Build history of the part. All positions in model axes, mm. Coordinates: 2 decimals unless noted, no trailing zeros. Write each loop counter-clockwise with the first axis right and the second up, starting at its lowest first coordinate (ties: lowest second). Pieces come first, ordered by that corner, then holes.
```python
from build123d import *

# Parameters (mm, degrees)
SKETCH1_W           = 288
SKETCH1_H           = 348
BOSS_EXTRUDE1_DEPTH = 25
SKETCH2_W           = 220
SKETCH2_H           = 25
SKETCH2_W_2         = 25
SKETCH2_H_2         = 280
CUT_EXTRUDE5_DEPTH  = 25


with BuildPart() as part:
    # Sketch1 → Boss-Extrude1 (new body)
    with BuildSketch(Plane(origin=(0, 0, 0), x_dir=(1, 0, 0), z_dir=(0, 1, 0))):
        with Locations((111.777306141, 159.011164947)):
            Rectangle(SKETCH1_W, SKETCH1_H)
    extrude(amount=BOSS_EXTRUDE1_DEPTH)

    # Sketch2 → Cut-Extrude5 (cut)
    with BuildSketch(Plane(origin=(0, 0, 0), x_dir=(1, 0, 0), z_dir=(0, 1, 0))):
        with Locations((111.777306141, 314.511164947)):
            Rectangle(SKETCH2_W, SKETCH2_H)
        with Locations((111.777306141, 3.511164947)):
            Rectangle(SKETCH2_W, SKETCH2_H)
        with Locations((237.277306141, 159.011164947)):
            Rectangle(SKETCH2_W_2, SKETCH2_H_2)
    extrude(amount=CUT_EXTRUDE5_DEPTH, mode=Mode.SUBTRACT)


solid = part.part
```
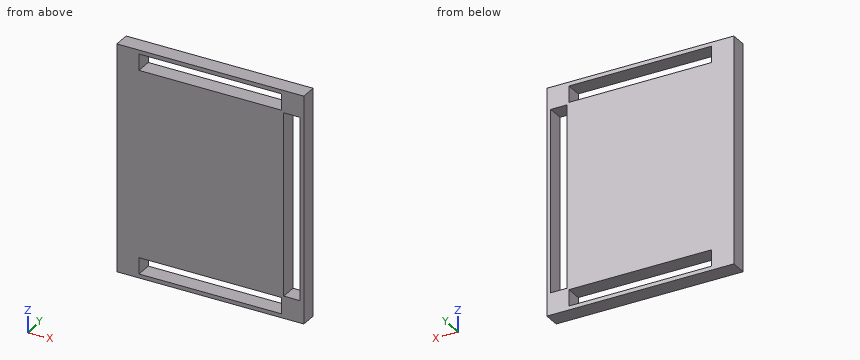
1. Saw through at B-B on y = 17.5. List the corners of the cut face in (x, z), plus the area to 3 significant figures.
Computed values:
outline: (-32.22, -333.01) - (255.78, -333.01) - (255.78, 14.99) - (-32.22, 14.99) - close; hole (1.78, -327.01) - (221.78, -327.01) - (221.78, -302.01) - (1.78, -302.01) - close; hole (1.78, -16.01) - (221.78, -16.01) - (221.78, 8.99) - (1.78, 8.99) - close; hole (224.78, -299.01) - (249.78, -299.01) - (249.78, -19.01) - (224.78, -19.01) - close
area: 82,200 mm2
2. Probe line 1 along Z through (x, y) = (92.5, 19); line 2 along X through (y, z) = (19.75, -130.5); line 3 along Z through (x, y) = (226.5, 8.5). List the from-to ranges inside material, lowest first.
Computed values:
line 1: z = -333.01 to -327.01, -302.01 to -16.01, 8.99 to 14.99
line 2: x = -32.22 to 224.78, 249.78 to 255.78
line 3: z = -333.01 to -299.01, -19.01 to 14.99
3. Saw through at C-C on z = -64. List the corners of the cut face in (x, y).
Computed values:
outline: (-32.22, 0) - (224.78, 0) - (224.78, 25) - (-32.22, 25) - close; (249.78, 0) - (255.78, 0) - (255.78, 25) - (249.78, 25) - close
4. Saw through at A-A on x = 61.5. List the corners of the cut face in (y, z), plus the area to 3 significant figures.
Computed values:
outline: (0, -333.01) - (25, -333.01) - (25, -327.01) - (0, -327.01) - close; (0, -302.01) - (25, -302.01) - (25, -16.01) - (0, -16.01) - close; (0, 8.99) - (25, 8.99) - (25, 14.99) - (0, 14.99) - close
area: 7,450 mm2
